```python
from build123d import *

# Parameters (mm, degrees)
ESQUISSE1_R             = 14
BOSS_EXTRU_1_DEPTH      = 19
ESQUISSE2_W             = 42
ESQUISSE2_H             = 7
ESQUISSE2_R             = 2.1
BOSS_EXTRU_2_DEPTH      = 0.8
CONG_1_R                = 3.5
ESQUISSE3_W             = 14.5
ESQUISSE3_H             = 8
BOSS_EXTRU_3_DEPTH      = 16.3
CONG_2_R                = 2
ESQUISSE4_R             = 4.6
BOSS_EXTRU_4_DEPTH      = 1.5
ESQUISSE5_R             = 2.5
BOSS_EXTRU_5_DEPTH      = 8.5
ESQUISSE6_W             = 12.644639
ESQUISSE6_H             = 4.455106
ESQUISSE6_W_2           = 15.068741
ESQUISSE6_H_2           = 4.782687
ENL_V_MAT_EXTRU_1_DEPTH = 6
ENL_V_START             = -1
ENL_V_MAT_EXTRU_2_DEPTH = 1
ENL_V_START_2           = -18.5
ESQUISSE8_R             = 2.5
ENL_V_MAT_EXTRU_3_DEPTH = 18.5


with BuildPart() as part:
    # Esquisse1 → Boss.-Extru.1 (new body)
    with BuildSketch(Plane(origin=(0, 0, 0), x_dir=(1, 0, 0), z_dir=(0, 1, 0))):
        with Locations(Location((0, 0, 0), (0, 0, 270))):
            Circle(ESQUISSE1_R)
    extrude(amount=BOSS_EXTRU_1_DEPTH)

    # Esquisse2 → Boss.-Extru.2 (add)
    with BuildSketch(Plane(origin=(0, 19, 0), x_dir=(1, 0, 0), z_dir=(0, 1, 0))):
        Rectangle(ESQUISSE2_W, ESQUISSE2_H)
        with Locations(Location((-17.5, 0, 0), (0, 0, 270))):
            Circle(ESQUISSE2_R, mode=Mode.SUBTRACT)
        with Locations(Location((17.5, 0, 0), (0, 0, 270))):
            Circle(ESQUISSE2_R, mode=Mode.SUBTRACT)
    extrude(amount=-BOSS_EXTRU_2_DEPTH)

    # Congé1
    cong_1_edges = [part.edges().sort_by_distance(p)[0] for p in [
        (21, 18.6, 3.5),
        (21, 18.6, -3.5),
        (-21, 18.6, 3.5),
        (-21, 18.6, -3.5),
    ]]
    fillet(cong_1_edges, radius=CONG_1_R - 0.0001)  # a hair under: the kernel refuses the full size

    # Esquisse3 → Boss.-Extru.3 (add)
    with BuildSketch(Plane(origin=(0, 19, 0), x_dir=(1, 0, 0), z_dir=(0, 1, 0))):
        with Locations((0, -13.5)):
            Rectangle(ESQUISSE3_W, ESQUISSE3_H)
    extrude(amount=-BOSS_EXTRU_3_DEPTH)

    # Congé2
    cong_2_edges = [part.edges().sort_by_distance(p)[0] for p in [
        (-7.25, 10.85, 17.5),
        (7.25, 10.85, 17.5),
    ]]
    fillet(cong_2_edges, radius=CONG_2_R)

    # Esquisse4 → Boss.-Extru.4 (add)
    with BuildSketch(Plane(origin=(0, 19, 0), x_dir=(1, 0, 0), z_dir=(0, 1, 0))):
        with Locations(Location((0, 8, 0), (0, 0, 270))):
            Circle(ESQUISSE4_R)
    extrude(amount=BOSS_EXTRU_4_DEPTH)

    # Esquisse5 → Boss.-Extru.5 (add)
    with BuildSketch(Plane(origin=(0, 20.5, 0), x_dir=(1, 0, 0), z_dir=(0, 1, 0))):
        with Locations(Location((0, 8, 0), (0, 0, 270))):
            Circle(ESQUISSE5_R)
    extrude(amount=BOSS_EXTRU_5_DEPTH)

    # Esquisse6 → Enlèv. mat.-Extru.1 (cut)
    with BuildSketch(Plane(origin=(0, 29, 0), x_dir=(1, 0, 0), z_dir=(0, 1, 0))):
        with Locations((0.098275, 11.727553)):
            Rectangle(ESQUISSE6_W, ESQUISSE6_H)
        with Locations((0.065517, 4.108657)):
            Rectangle(ESQUISSE6_W_2, ESQUISSE6_H_2)
    extrude(amount=-ENL_V_MAT_EXTRU_1_DEPTH, mode=Mode.SUBTRACT)

    # Esquisse7 → Enlèv. mat.-Extru.2 (cut)
    with BuildSketch(Plane(origin=(0, 19, 0), x_dir=(1, 0, 0), z_dir=(0, 1, 0)).offset(ENL_V_START)):
        with BuildLine():
            Line((-7.25, -11.97654), (-7.25, -22.169225))
            Line((-7.25, -22.169225), (7.25, -22.169225))
            Line((7.25, -22.169225), (7.25, -11.97654))
            ThreePointArc((7.25, -11.97654), (0, -14), (-7.25, -11.97654))
        make_face()
    extrude(amount=ENL_V_MAT_EXTRU_2_DEPTH, mode=Mode.SUBTRACT)

    # Esquisse8 → Enlèv. mat.-Extru.3 (cut)
    with BuildSketch(Plane(origin=(0, 29, 0), x_dir=(1, 0, 0), z_dir=(0, 1, 0)).offset(ENL_V_START_2)):
        with Locations(Location((0, 8, 0), (0, 0, 270))):
            Circle(ESQUISSE8_R)
    extrude(amount=ENL_V_MAT_EXTRU_3_DEPTH, mode=Mode.SUBTRACT)


solid = part.part
```
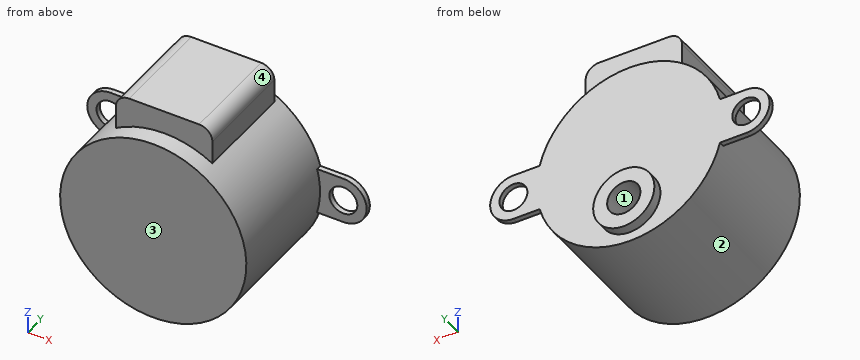
The listing builds one solid part. Answer for the finished solid, in the listing's coordinates (mm). Face numbers are marked on the shaded views. Round coordinates to 2 decimals unless told otherwise and drop trailing zeros. Order: outer loops, then holes, each group sorted by start corner. A loop starts at its lowest first (then second) coordinate and runs counter-clockwise, first axis right, second up. Notation, with made-up numbers: (69, 60.25) - (97, 60.25) arc R32 ccw to (97, 92.25) - close; hole circle Ø9 at (79.5, -4.5). An arc over 180 degrees is marked (long way). Put each result on its own line as item: value. Start each with the question number.
(1) Determine the mould class of the marked faces 1, 2, 3 and 4 for opening direction X: released by +X, released by -X, zero draft, split by the parting line, or undercut.
(2) Find section A-A (y = 16.25). Give the vertices of the cut face in (x, z).
(3) Find section C-C (z = -8). Give the vertices of the cut face in (x, y).
(4) Find section D-D (x = -9.5). Give the vertices of the cut face in (y, z), plus the area to 3 significant figures.
(5) Straight lines are drawn through the part: probe 1 along X at (y, z) = (18.55, 0); probe 2 along X at (y, z) = (18, 3.5); probe 3 along Y at (x, z) = (4, 7). For each, find the intervals that lie inside material, in ascending order. Write a range as from..to.
(6) Given P1, Ø5, axis at y = 4, z = -2.5, coming from the +X side; P2, Ø1.1, axis at y = 14.5, z = 13, coming from the +X side; P3, Ø1, axis at y = 6, z = 2, coming from the +X side, each flat-ended and moving along its own axis, determine where each tip first touches the part or whether it passes through.
(7) Find section B-B (x = 0). Give the vertices of the cut face in (y, z), plus the area to 3 significant figures.
Reply:
1. face 1: undercut
1. face 2: split by the parting line
1. face 3: zero draft
1. face 4: released by +X
2. outline: (-7.25, 11.98) arc R14 ccw (long way) to (7.25, 11.98) - (7.25, 15.5) arc R2 ccw to (5.25, 17.5) - (-5.25, 17.5) arc R2 ccw to (-7.25, 15.5) - close; hole circle Ø5 at (0, -8)
3. outline: (-11.49, 0) - (11.49, 0) - (11.49, 19) - (4.6, 19) - (4.6, 20.5) - (2.5, 20.5) - (2.5, 10.5) - (-2.5, 10.5) - (-2.5, 20.5) - (-4.6, 20.5) - (-4.6, 19) - (-11.49, 19) - close
4. outline: (0, -10.28) - (19, -10.28) - (19, 10.28) - (0, 10.28) - close
4. area: 391 mm^2
5. probe 1: -21..-19.6, -15.4..15.4, 19.6..21
5. probe 2: -13.56..13.56
5. probe 3: 0..19
6. P1: x = 14
6. P2: x = 7.25
6. P3: x = 13.92
7. outline: (0, -14) - (19, -14) - (19, -12.6) - (20.5, -12.6) - (20.5, -10.5) - (10.5, -10.5) - (10.5, -5.5) - (20.5, -5.5) - (20.5, -3.4) - (19, -3.4) - (19, 14) - (18, 14) - (18, 17.5) - (2.7, 17.5) - (2.7, 14) - (0, 14) - close
7. area: 549 mm^2
